Check sheet for the drawn part. Datum: minimum x, y, z corner. Units: mm. A direction names the side the tool comes from. Give positions to 0.01 mm unless a question says otherwise; leave off trailing zeros. Order: outer loops, then holes, each group sorted by start corner. A loop starts at its lowest first (then second) coordinate and runs counter-clockwise, first axis right, second up. Notation, with made-up numbers: (-29.5, 40) - (-6.5, 40) arc R23 cw to (-6.5, 74) - close; hole circle Ø10 at (61.5, 45). An arc over 180 degrees is marked (long way). Answer as a JSON object with one key per item and string values. Group by question number.
(1) Depth check by flat-ended pin: pin 1 Ø4.5 at (x, y) = (7.5, 12.5) entering from -Z; pin 2 Ø1 at (x, z) = (59, 6) entering from -Y; pin 3 Ø2.5 at (x, y) = (52.5, 12.5) entering from -Z; pin 4 Ø5 at (y, z) = (13.5, 4) entering from -X. Enter the tip coordinate at first touch or a pass-through.
(2) Access from +Z, -Z, +X, -X, +Y, -Y to the whole of each face (thin tool, end or side, straight path). Record for the marked faces 1 and 2.
(3) Section check A-A (y = 12.5). Record the boundary of the cut face in (x, z).
(4) Section check D-D (y = 15.5). Record the boundary of the cut face in (x, z).
(5) Section check C-C (z = 15). Record the boundary of the cut face in (x, y), then the cut area to 3 significant figures.
(6) Section check B-B (x = 17.5). Record the boundary of the cut face in (y, z).
(7) Thickness scan on line 1 (X direction, y = 12.5, z = 2.75); line 2 (Y direction, x = 67.5, z = 11.5); line 3 (X direction, y = 11.5, z = 8). Record the ranges inside material, lowest first.
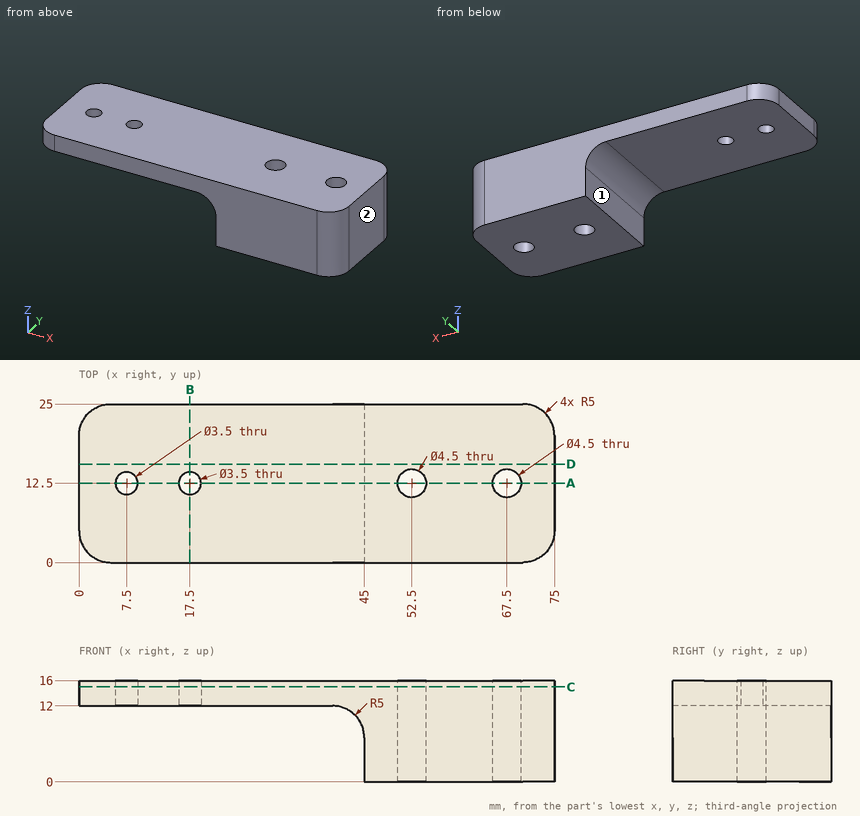
Solutions:
{
 "1": {"pin 1": "stops at z = 12", "pin 2": "stops at y = 0", "pin 3": "passes through", "pin 4": "stops at x = 45"},
 "2": {"face 1": "-Z, -X, +Y, -Y", "face 2": "+Z, -Z, +X, +Y, -Y"},
 "3": {"outline": "(0, 12) - (5.75, 12) - (5.75, 16) - (0, 16) - close; (9.25, 12) - (15.75, 12) - (15.75, 16) - (9.25, 16) - close; (19.25, 12) - (40, 12) arc R5 cw to (45, 7) - (45, 0) - (50.25, 0) - (50.25, 16) - (19.25, 16) - close; (54.75, 0) - (65.25, 0) - (65.25, 16) - (54.75, 16) - close; (69.75, 0) - (75, 0) - (75, 16) - (69.75, 16) - close"},
 "4": {"outline": "(0, 12) - (40, 12) arc R5 cw to (45, 7) - (45, 0) - (75, 0) - (75, 16) - (0, 16) - close"},
 "5": {"outline": "(0, 5) arc R5 ccw to (5, 0) - (70, 0) arc R5 ccw to (75, 5) - (75, 20) arc R5 ccw to (70, 25) - (5, 25) arc R5 ccw to (0, 20) - close; hole circle Ø3.5 at (7.5, 12.5); hole circle Ø3.5 at (17.5, 12.5); hole circle Ø4.5 at (52.5, 12.5); hole circle Ø4.5 at (67.5, 12.5)", "area": "1,800 mm2"},
 "6": {"outline": "(0, 12) - (10.75, 12) - (10.75, 16) - (0, 16) - close; (14.25, 12) - (25, 12) - (25, 16) - (14.25, 16) - close"},
 "7": {"line 1": "x = 45 to 50.25, 54.75 to 65.25, 69.75 to 75", "line 2": "y = 0 to 10.25, 14.75 to 25", "line 3": "x = 44.9 to 50.48, 54.52 to 65.48, 69.52 to 75"}
}
